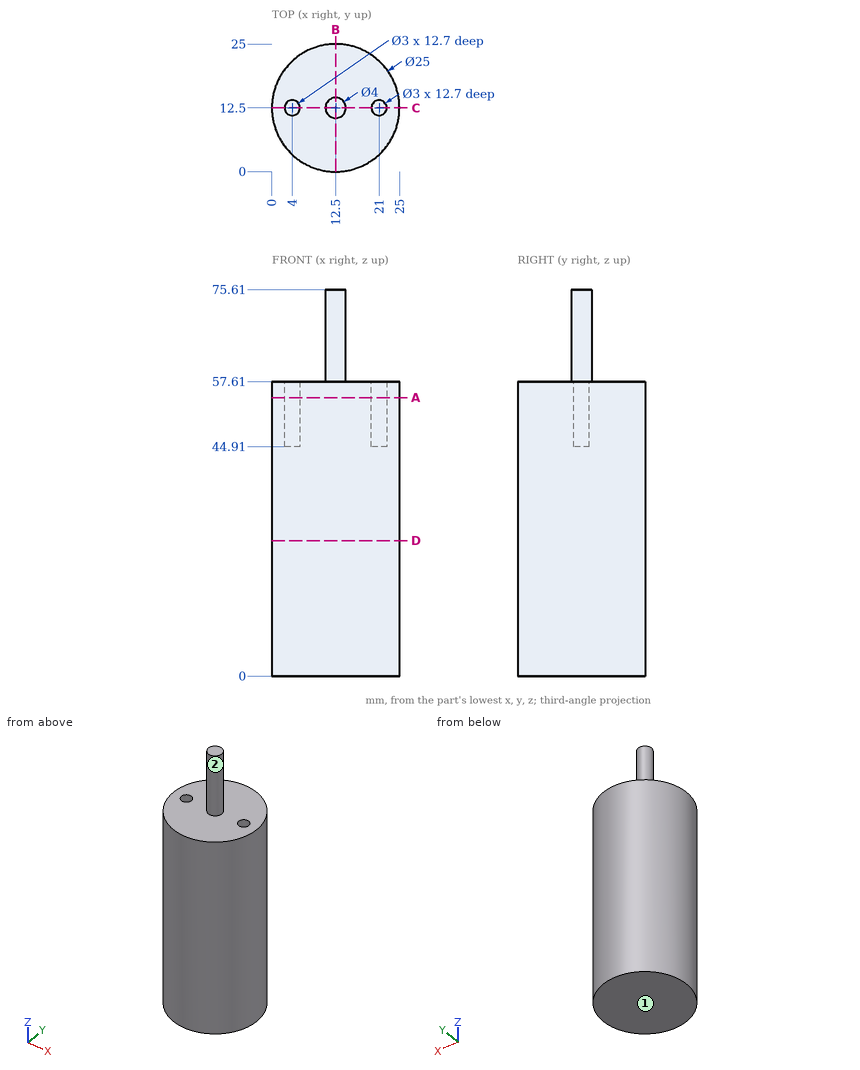
Source: three-view drawing plus pictorial views. Frame: mm from the lowest corner of the part. A direction names the side the tool comes from. Round coordinates to 2 decimals unless told otherwise and drop trailing zeros. Write each loop counter-clockwise with the first axis right and the second up, starting at its lowest first coordinate (ties: lowest second). Pieces come first, ordered by that corner, then holes. Notation, with made-up numbers: M 21.25,43 L 51.25,43 A20 ccw 51.25,48 Z; hole C 27,11 d11. An arc over 180 degrees is marked long. One line per item, written item: value. Start each with the question number.
Item 1: Section query B-B (x = 12.5). Return the cut outline in (y, z).
Item 2: Section query C-C (y = 12.5). Return the cut outline in (x, z), plus the area to 3 significant figures.
Item 3: Pin query (flat end, axial travel): pin 1 (1 mm diameter, centred on x = 13.5, z = 39, fed in from +Y); pin 2 (5 mm diameter, centred on x = 21.5, z = 13.5, fed in from -Y); pin 3 (2.5 mm diameter, centred on x = 20.5, y = 12, fed in from +Z). Return the tip coordinate at first contact, or that it passes through.
Item 4: Ray query, L1, parallel to X at y = 13.5, z = 51.5; L2, parallel to Z at x = 21.5, y = 16.5; L3, parallel to Y at x = 4, z = 50. Return the intervals inside material, ascending. Write a range as from..to.
Item 5: Section query D-D (z = 26.5). Return the cut outline in (x, y).
Item 6: Section query A-A (z = 54.5). Return the cut outline in (x, y).
Item 7: Set-up query: the marked faces 1 and 2. Return all of +Z, -Z, +X, -X, +Y, -Y with unobstructed straight access to the full face (end or side cutting, diameter ignored); none if empty.
Result set:
1. outline: M 0,0 L 25,0 L 25,57.61 L 14.5,57.61 L 14.5,75.61 L 10.5,75.61 L 10.5,57.61 L 0,57.61 Z
2. outline: M 0,0 L 25,0 L 25,57.61 L 22.5,57.61 L 22.5,44.91 L 19.5,44.91 L 19.5,57.61 L 14.5,57.61 L 14.5,75.61 L 10.5,75.61 L 10.5,57.61 L 5.5,57.61 L 5.5,44.91 L 2.5,44.91 L 2.5,57.61 L 0,57.61 Z
2. area: 1,440 mm²
3. pin 1: stops at y = 24.99
3. pin 2: stops at y = 1.82
3. pin 3: stops at z = 57.61
4. L1: x = 0.04..2.88, 5.12..19.88, 22.12..24.96
4. L2: z = 0..57.61
4. L3: y = 3.33..11, 14..21.67
5. outline: C 12.5,12.5 d25
6. outline: C 12.5,12.5 d25; hole C 4,12.5 d3; hole C 21,12.5 d3
7. face 1: -Z, +X, -X, +Y, -Y
7. face 2: +Z
